Autodesk Inventor part; units mm, degrees
ref_plane "YZ Plane" through (0, 0, 0) normal (1, 0, 0) x (0, 1, 0)
ref_plane "XZ Plane" through (0, 0, 0) normal (0, 1, 0) x (-1, 0, 0)
ref_plane "XY Plane" through (0, 0, 0) normal (0, 0, 1) x (1, 0, 0)
sketch "Эскиз1" plane through (0, 0, 0) normal (0, 1, 0) x (-1, 0, 0)
  line L0 (-16, 7) -> (16, 7)
  line L1 (16, 7) -> (16, -7)
  line L2 (16, -7) -> (-16, -7)
  line L3 (-16, -7) -> (-16, 7)
  line L4 (-16, 7) -> (16, -7) construction
  line L5 (16, 7) -> (-16, -7) construction
  point P0 (0, 0)
  dimension "d0" = 32
  dimension "d1" = 14
extrude "Выдавливание1" add sketch "Эскиз1" along normal blind 1.3
sketch "Эскиз4" plane through (0, 1.3, 0) normal (0, 1, 0) x (1, 0, 0)
  line L0 (-16, -7) -> (16, -7)
  line L1 (16, -7) -> (16, -6.5)
  line L2 (16, -7) -> (16, 7)
  line L3 (16, -6.5) -> (15.9, -6.5)
  line L4 (15.9, -6.5) -> (9.9, -6.5)
  line L5 (9.9, -6.5) -> (9.9, 6.5)
  line L6 (9.9, 6.5) -> (15.9, 6.5)
  line L7 (15.9, 6.5) -> (15.9, -6.5)
  point P0 (0, 0)
  dimension "d13" = 0.5
  dimension "d14" = 0.1
  dimension "d15" = 6
  dimension "d16" = 13
extrude "Выдавливание4" add sketch "Эскиз4" along normal blind 10
sketch "Эскиз5" plane through (0, 11.3, 0) normal (0, 1, 0) x (1, 0, 0)
  line L0 (9.9, 6.5) -> (9.9, -6.5)
  line L1 (15.9, -2.5) -> (9.9, -2.5)
  line L2 (9.9, -2.5) -> (9.9, 2.5)
  line L3 (9.9, 2.5) -> (15.9, 2.5)
  line L4 (15.9, 2.5) -> (15.9, -2.5)
  line L5 (15.9, -2.5) -> (9.9, 2.5) construction
  line L6 (9.9, -2.5) -> (15.9, 2.5) construction
  point P0 (0, 0)
  point P1 (12.9, 0)
  dimension "d19" = 5
extrude "Выдавливание5" cut sketch "Эскиз5" against normal blind 8
sketch "Эскиз6" plane through (0, 1.3, 0) normal (0, 1, 0) x (1, 0, 0)
  line L0 (-16, 7) -> (-16, -7)
  line L1 (-16, 0) -> (-10, 0)
  line L2 (-10, 0) -> (-7, 0)
  circle A0 centre (-8.5, 0) radius 1.5
  point P0 (0, 0)
  dimension "d22" = 6
  dimension "d23" = 3
extrude "Выдавливание6" cut sketch "Эскиз6" against normal blind 8
sketch "Эскиз10" plane through (0, 1.3, 0) normal (0, 1, 0) x (1, 0, 0)
  line L0 (2.3, 6) -> (-1.7, 6)
  line L1 (-1.7, 6) -> (-1.7, 1)
  line L2 (-1.7, 1) -> (2.3, 1)
  line L3 (2.3, 1) -> (2.3, 6)
  line L4 (-12.7, 2.9) -> (-12.7, 4.9)
  line L5 (16, 7) -> (-16, 7)
  point P0 (0, 0)
  dimension "d49" = 4
  dimension "d50" = 5
  dimension "d51" = 11
  dimension "d52" = 1
extrude "Выдавливание9" add sketch "Эскиз10" along normal blind 1.8
chamfer "Фаска1" distance 0.25 angle 45 4 edges at (-1.7, 3.1, -3.5) (0.3, 3.1, -1) (2.3, 3.1, -3.5) (0.3, 3.1, -6)
sketch "Эскиз11" plane through (0, 1.3, 0) normal (0, 1, 0) x (1, 0, 0)
  line L0 (-1.7, 1) -> (-1.7, 6)
  line L1 (-1.7, 6) -> (-1.7, 5.8)
  line L2 (-1.7, 5.8) -> (-2.7, 5.8)
  line L3 (-2.7, 5.8) -> (-2.7, 5.3)
  line L4 (-2.7, 5.3) -> (-1.7, 5.3)
  line L5 (-1.7, 5.3) -> (-1.7, 5.8)
  line L6 (-1.7, 4.7) -> (-1.7, 4.5)
  line L7 (-1.7, 4.5) -> (-2.7, 4.5)
  line L8 (-2.7, 4.5) -> (-2.7, 4)
  line L9 (-2.7, 4) -> (-1.7, 4)
  line L10 (-1.7, 4) -> (-1.7, 4.5)
  line L11 (-1.7, 3.4) -> (-1.7, 3.2)
  line L12 (-1.7, 3.2) -> (-2.7, 3.2)
  line L13 (-2.7, 3.2) -> (-2.7, 2.7)
  line L14 (-2.7, 2.7) -> (-1.7, 2.7)
  line L15 (-1.7, 2.7) -> (-1.7, 3.2)
  line L16 (-1.7, 2.1) -> (-1.7, 1.9)
  line L17 (-1.7, 1.9) -> (-2.7, 1.9)
  line L18 (-2.7, 1.9) -> (-2.7, 1.4)
  line L19 (-2.7, 1.4) -> (-1.7, 1.4)
  line L20 (-1.7, 1.4) -> (-1.7, 1.9)
  line L21 (-1.7, 6) -> (2.3, 6)
  line L22 (0.3, 6) -> (0.3, 4.6)
  line L23 (2.3, 1) -> (2.3, 6)
  line L24 (2.3, 6) -> (2.3, 5.8)
  line L25 (2.3, 5.8) -> (3.3, 5.8)
  line L26 (3.3, 5.8) -> (3.3, 5.3)
  line L27 (3.3, 5.3) -> (2.3, 5.3)
  line L28 (2.3, 5.3) -> (2.3, 5.8)
  line L29 (2.3, 4.7) -> (2.3, 4.5)
  line L30 (2.3, 4.5) -> (3.3, 4.5)
  line L31 (3.3, 4.5) -> (3.3, 4)
  line L32 (3.3, 4) -> (2.3, 4)
  line L33 (2.3, 4) -> (2.3, 4.5)
  line L34 (2.3, 3.4) -> (2.3, 3.2)
  line L35 (2.3, 3.2) -> (3.3, 3.2)
  line L36 (3.3, 3.2) -> (3.3, 2.7)
  line L37 (3.3, 2.7) -> (2.3, 2.7)
  line L38 (2.3, 2.7) -> (2.3, 3.2)
  line L39 (2.3, 2.1) -> (2.3, 1.9)
  line L40 (2.3, 1.9) -> (3.3, 1.9)
  line L41 (3.3, 1.9) -> (3.3, 1.4)
  line L42 (3.3, 1.4) -> (2.3, 1.4)
  line L43 (2.3, 1.4) -> (2.3, 1.9)
  point P0 (0, 0)
  dimension "d58" = 0.2
  dimension "d59" = 1
  dimension "d60" = 0.5
  dimension "d63" = 1.3
extrude "Выдавливание10" add sketch "Эскиз11" along normal blind 1
chamfer "Фаска2" distance 0.75 angle 45 8 edges at (-2.7, 2.3, -5.55) (-2.7, 2.3, -4.25) (-2.7, 2.3, -2.95) (-2.7, 2.3, -1.65) (3.3, 2.3, -1.65) (3.3, 2.3, -2.95) (3.3, 2.3, -4.25) (3.3, 2.3, -5.55)
sketch "Эскиз18" plane through (0, 0, 0) normal (0, -1, 0) x (1, 0, 0)
  line L0 (16, 7) -> (-16, 7)
  line L1 (-16, 7) -> (-15.3, 7)
  line L2 (-15.3, 7) -> (-15.3, 5.2)
  line L3 (-15, 5.2) -> (-13, 5.2)
  line L4 (-12.7, 4.9) -> (-12.7, 2.9)
  line L5 (-13, 2.6) -> (-15, 2.6)
  line L6 (-15.3, 2.9) -> (-15.3, 4.9)
  arc A0 (-12.7, 4.9) -> (-13, 5.2) centre (-13, 4.9) ccw
  arc A1 (-13, 2.6) -> (-12.7, 2.9) centre (-13, 2.9) ccw
  arc A2 (-15.3, 2.9) -> (-15, 2.6) centre (-15, 2.9) ccw
  arc A3 (-15, 5.2) -> (-15.3, 4.9) centre (-15, 4.9) ccw
  line L7 (-15.3, 4.4) -> (-15.3, 2.6)
  arc A4 (-15, 2.6) -> (-15.3, 2.3) centre (-15, 2.3) ccw
  line L8 (-15, 2.6) -> (-13, 2.6)
  arc A5 (-12.7, 2.3) -> (-13, 2.6) centre (-13, 2.3) ccw
  line L9 (-15.3, 0.3) -> (-15.3, 2.3)
  arc A6 (-15.3, 0.3) -> (-15, 0) centre (-15, 0.3) ccw
  line L10 (-12.7, 2.3) -> (-12.7, 0.3)
  arc A7 (-13, 0) -> (-12.7, 0.3) centre (-13, 0.3) ccw
  line L11 (-13, 0) -> (-15, 0)
  line L12 (-15.3, 1.8) -> (-15.3, 0)
  arc A8 (-15, 0) -> (-15.3, -0.3) centre (-15, -0.3) ccw
  line L13 (-15, 0) -> (-13, 0)
  arc A9 (-12.7, -0.3) -> (-13, 0) centre (-13, -0.3) ccw
  line L14 (-15.3, -2.3) -> (-15.3, -0.3)
  arc A10 (-15.3, -2.3) -> (-15, -2.6) centre (-15, -2.3) ccw
  line L15 (-12.7, -0.3) -> (-12.7, -2.3)
  arc A11 (-13, -2.6) -> (-12.7, -2.3) centre (-13, -2.3) ccw
  line L16 (-13, -2.6) -> (-15, -2.6)
  line L17 (-15.3, -0.8) -> (-15.3, -2.6)
  arc A12 (-15, -2.6) -> (-15.3, -2.9) centre (-15, -2.9) ccw
  line L18 (-15, -2.6) -> (-13, -2.6)
  arc A13 (-12.7, -2.9) -> (-13, -2.6) centre (-13, -2.9) ccw
  line L19 (-15.3, -4.9) -> (-15.3, -2.9)
  arc A14 (-15.3, -4.9) -> (-15, -5.2) centre (-15, -4.9) ccw
  line L20 (-12.7, -2.9) -> (-12.7, -4.9)
  arc A15 (-13, -5.2) -> (-12.7, -4.9) centre (-13, -4.9) ccw
  line L21 (-13, -5.2) -> (-15, -5.2)
  point P0 (0, 0)
  point P1 (-12.7, 2.6)
  point P2 (-12.7, 5.2)
  point P3 (-12.7, 2.6)
  point P4 (-12.7, 0)
  point P5 (-12.7, 0)
  point P6 (-12.7, -2.6)
  point P7 (-12.7, -2.6)
  point P8 (-15.3, -5.2)
  point P9 (-12.7, -5.2)
  dimension "d105" = 0.7
  dimension "d106" = 1.8
  dimension "d107" = 2.6
  dimension "d108" = 2.6
  dimension "d109" = 0.3
  dimension "d112" = 2.6
extrude "Выдавливание11" add sketch "Эскиз18" along normal blind 2.5
sketch "Эскиз19" plane through (0, -2.5, 0) normal (0, -1, 0) x (1, 0, 0)
  line L0 (-15, 5.2) -> (-13, 5.2)
  line L1 (-14, 5.2) -> (-14, 3.9)
  line L2 (-14.4, 3.5) -> (-13.6, 3.5)
  line L3 (-13.6, 3.5) -> (-13.6, 4.3)
  line L4 (-13.6, 4.3) -> (-14.4, 4.3)
  line L5 (-14.4, 4.3) -> (-14.4, 3.5)
  line L6 (-14.4, 3.5) -> (-13.6, 4.3) construction
  line L7 (-13.6, 3.5) -> (-14.4, 4.3) construction
  line L8 (-14.4, 0.9) -> (-13.6, 0.9)
  line L9 (-13.6, 0.9) -> (-13.6, 1.7)
  line L10 (-13.6, 1.7) -> (-14.4, 1.7)
  line L11 (-14.4, 1.7) -> (-14.4, 0.9)
  line L12 (-14.4, 0.9) -> (-13.6, 1.7) construction
  line L13 (-13.6, 0.9) -> (-14.4, 1.7) construction
  line L14 (-14.4, -1.7) -> (-13.6, -1.7)
  line L15 (-13.6, -1.7) -> (-13.6, -0.9)
  line L16 (-13.6, -0.9) -> (-14.4, -0.9)
  line L17 (-14.4, -0.9) -> (-14.4, -1.7)
  line L18 (-14.4, -1.7) -> (-13.6, -0.9) construction
  line L19 (-13.6, -1.7) -> (-14.4, -0.9) construction
  line L20 (-14.4, -4.3) -> (-13.6, -4.3)
  line L21 (-13.6, -4.3) -> (-13.6, -3.5)
  line L22 (-13.6, -3.5) -> (-14.4, -3.5)
  line L23 (-14.4, -3.5) -> (-14.4, -4.3)
  line L24 (-14.4, -4.3) -> (-13.6, -3.5) construction
  line L25 (-13.6, -4.3) -> (-14.4, -3.5) construction
  point P0 (0, 0)
  point P1 (-14, 1.3)
  point P2 (-14, -1.3)
  point P3 (-14, -3.9)
  dimension "d119" = 1.3
  dimension "d120" = 0.8
  dimension "d121" = 0.8
  dimension "d124" = 2.6
extrude "Выдавливание12" add sketch "Эскиз19" along normal blind 6
properties part number "Оптический датчик"
The listing builds one solid part. Answer for the finished solid, in the listing's coordinates (mm). A direction names the side the tool comes from. Coordinates: 2 decimals unless noted, no trailing zeros. Write each loop counter-clockwise with the first axis right and the second up, starting at its lowest first coordinate (ties: lowest second). Pieces come first, ordered by that corner, then holes. Notation, with made-up numbers: (40, 2) - (80, 2) arc R26 ccw to (80, 30) - close; hole circle Ø10 at (-28, -26.75). An arc over 180 degrees is marked (long way). Return JSON: item names as keys, results as strings. Group by question number.
1. A cutting plane is placed at C-C, the plane x = 9.5. Determine the outline of the cut face in (y, z), plus the area to 3 significant figures.
2. Given pin 1 (5 mm diameter, centred on x = -7, z = 4.5, fed in from -Y); pin 2 (1.8 mm diameter, centred on x = 0, z = -4.5, fed in from +Y); pin 3 (0.9 mm diameter, centred on y = -5.5, z = 4, fed in from -X); pin 4 (2 mm diameter, centred on y = -0.5, z = -2.5, fed in from -X), each flat-ended and moving along its own axis, determine where each tip first touches the part or whether it passes through.
3. A cutting plane is placed at A-A, the plane x = -8.5. Determine the outline of the cut face in (y, z), plus the area to 3 significant figures.
4. Which of the six approach directions +Z, -Z, +X, -X, +Y, -Y give full straight-line access (tool end or side, diameter ignored) to faces 1 (the flat face through (13, 3.3, 0)), 2 (the flat face through (-14, -5, 0.9)), 3 (the flat face through (0, 3.1, -4)), 4 (the flat face through (-12.7, -1, 4)), 5 (the flat face through (15.9, 6, -3))?
5. A cutting plane is placed at B-B, the plane y = -1.75. Determine the outline of the cut face in (x, z).
6. Straight lines are drawn through the part: L1, parallel to Z at x = -8.5, y = 1.05; L2, parallel to X at y = 0.9, z = 0; L3, parallel to Y at x = -4.5, z = 6. For each, find the intervals that lie inside material, in ascending order.
7. Determine the mould class of faces 6 (the flat face through (-14, -5, -0.9)), 7 (the flat face through (-12.7, -1, 1)), 8 (the flat face through (2.3, 2.2, -3.5)), 9 (the flat face through (-15.3, -1, 4)) for opening direction X: released by +X, released by -X, zero draft, split by the parting line, or undercut.
Ans:
{
 "1": {"outline": "(0, -7) - (1.3, -7) - (1.3, 7) - (0, 7) - close", "area": "18.2 mm²"},
 "2": {"pin 1": "y = 0", "pin 2": "y = 3.1", "pin 3": "x = -14.4", "pin 4": "x = -16"},
 "3": {"outline": "(0, -7) - (1.3, -7) - (1.3, -1.5) - (0, -1.5) - close; (0, 1.5) - (1.3, 1.5) - (1.3, 7) - (0, 7) - close", "area": "14.3 mm²"},
 "4": {"face 1": "+X, -X, +Y", "face 2": "+X, -X, -Y", "face 3": "+Z, -Z, -X, +Y", "face 4": "+Z, -Z, +X, -Y", "face 5": "+Z, -Z, +X, +Y"},
 "5": {"outline": "(-15.3, -4.9) arc R0.3 ccw to (-15, -5.2) - (-13, -5.2) arc R0.3 ccw to (-12.7, -4.9) - (-12.7, -2.9) arc R0.3 ccw to (-13, -2.6) arc R0.3 ccw to (-12.7, -2.3) - (-12.7, -0.3) arc R0.3 ccw to (-13, 0) arc R0.3 ccw to (-12.7, 0.3) - (-12.7, 2.3) arc R0.3 ccw to (-13, 2.6) arc R0.3 ccw to (-12.7, 2.9) - (-12.7, 4.9) arc R0.3 ccw to (-13, 5.2) - (-15, 5.2) arc R0.3 ccw to (-15.3, 4.9) - (-15.3, 2.9) arc R0.3 ccw to (-15, 2.6) arc R0.3 ccw to (-15.3, 2.3) - (-15.3, 0.3) arc R0.3 ccw to (-15, 0) arc R0.3 ccw to (-15.3, -0.3) - (-15.3, -2.3) arc R0.3 ccw to (-15, -2.6) arc R0.3 ccw to (-15.3, -2.9) - close"},
 "6": {"L1": "-7 to -1.5, 1.5 to 7", "L2": "-16 to -10, -7 to 16", "L3": "0 to 1.3"},
 "7": {"face 6": "zero draft", "face 7": "released by +X", "face 8": "undercut", "face 9": "released by -X"}
}
